```python
from build123d import *

# Parameters (mm, degrees)
SZKIC1_R                    = 2
DODANIE_WYCI_GNI_CIE1_DEPTH = 5
ZAOKR_GLENIE1_R             = 2
ZAOKR_GLENIE2_R             = 8


with BuildPart() as part:
    # Szkic1 → Dodanie-wyciągnięcie1 (new body)
    with BuildSketch(Plane.XY):
        with BuildLine():
            ThreePointArc((12, 0), (15, 3), (18, 0))
            Line((18, 0), (18, -15))
            Line((18, -15), (25, -15))
            Line((25, -15), (25, 15))
            Line((25, 15), (2, 15))
            Line((2, 15), (-2, 15))
            Line((-2, 15), (-25, 15))
            Line((-25, 15), (-25, -15))
            Line((-25, -15), (-18, -15))
            Line((-18, -15), (-18, 0))
            ThreePointArc((-18, 0), (-15, 3), (-12, 0))
            Line((-12, 0), (-12, -15))
            Line((-12, -15), (12, -15))
            Line((12, -15), (12, 0))
        make_face()
        with BuildLine():
            Line((-2, 15), (2, 15))
            Line((2, 15), (2, 20))
            ThreePointArc((2, 20), (0, 18), (-2, 20))
            Line((-2, 20), (-2, 15))
        make_face()
        with Locations((0, 20)):
            Circle(SZKIC1_R)
    extrude(amount=DODANIE_WYCI_GNI_CIE1_DEPTH)

    # Zaokrąglenie1
    zaokr_glenie1_edges = [part.edges().sort_by_distance(p)[0] for p in [
        (12, -15, 2.5),
        (-12, -15, 2.5),
        (-18, -15, 2.5),
        (-25, -15, 2.5),
        (-2, 15, 2.5),
        (2, 15, 2.5),
        (25, -15, 2.5),
        (18, -15, 2.5),
    ]]
    fillet(zaokr_glenie1_edges, radius=ZAOKR_GLENIE1_R)

    # Zaokrąglenie2
    zaokr_glenie2_edges = [part.edges().sort_by_distance(p)[0] for p in [
        (-25, 15, 2.5),
        (25, 15, 2.5),
    ]]
    fillet(zaokr_glenie2_edges, radius=ZAOKR_GLENIE2_R)


solid = part.part
```
Here's how the part is built. I have some questions about the finished solid (model axes, mm). A direction names the side the tool comes from. Give positions to 0.01 mm unless a question says otherwise; leave off trailing zeros. Order: outer loops, then holes, each group sorted by start corner. A loop starts at its lowest first (then second) coordinate and runs counter-clockwise, first axis right, second up. Notation, with made-up numbers: (-19.5, 12) - (-15.5, 12) arc R16 cw to (-15.5, 37) - close; hole circle Ø6 at (44, 61). An arc over 180 degrees is marked (long way). Answer as a JSON object with one key per item and string values. Group by question number.
Item 1: For P1, Ø2.5, axis at y = 18.5, z = 3, coming from the +X side; P2, Ø1.5, axis at x = -4.5, z = 1, coming from the +Y side; P3, Ø2, axis at x = -12.5, z = 2.5, coming from the -Y side, each with a flat end and sliding along its axis, tell me the tip position at first contact or that it passes through.
Item 2: If we section it at B-B on z = 2.1: Please give me the cut outline in (x, y), and give its area (3 significant figures).
Item 3: If we section it at D-D on x = -15: Please give me the cut outline in (y, z).
Item 4: If we section it at C-C on x = 6: Please give me the cut outline in (y, z), and give its area (3 significant figures).
Item 5: Please list where these lines run through material, in increasing order: probe 1 along X at (y, z) = (-10, 0.95); probe 2 along X at (y, z) = (2, 4.45); probe 3 along Y at (x, z) = (4.5, 2.85).
Item 6: Which directions (+Z, -Z, +X, -X, +Y, -Y) give clear straight access to the entire face, cutting with the end or side of a thin tool? Please do faces 1 (the flat face through (-12, -6, 2)), 2 (the flat face through (0, -15, 2)), 3 (the flat face through (-2, 19, 2)), 4 (the flat face through (2, 18, 2)).
Item 7: If we section it at A-A on y = -2.5: Please give me the cut outline in (x, z).
Result set:
{
 "1": {"P1": "x = 2", "P2": "y = 15.02", "P3": "y = -14.32"},
 "2": {"outline": "(-25, -13) arc R2 ccw to (-23, -15) - (-20, -15) arc R2 ccw to (-18, -13) - (-18, 0) arc R3 cw to (-12, 0) - (-12, -13) arc R2 ccw to (-10, -15) - (10, -15) arc R2 ccw to (12, -13) - (12, 0) arc R3 cw to (18, 0) - (18, -13) arc R2 ccw to (20, -15) - (23, -15) arc R2 ccw to (25, -13) - (25, 7) arc R8 ccw to (17, 15) - (4, 15) arc R2 cw to (2, 17) - (2, 20) arc R2 ccw to (-2, 20) - (-2, 17) arc R2 cw to (-4, 15) - (-17, 15) arc R8 ccw to (-25, 7) - close", "area": "1,290 mm²"},
 "3": {"outline": "(3, 0) - (15, 0) - (15, 5) - (3, 5) - close"},
 "4": {"outline": "(-15, 0) - (15, 0) - (15, 5) - (-15, 5) - close", "area": "150 mm²"},
 "5": {"probe 1": "-25 to -18, -12 to 12, 18 to 25", "probe 2": "-25 to -17.24, -12.76 to 12.76, 17.24 to 25", "probe 3": "-15 to 15"},
 "6": {"face 1": "+Z, -Z, -Y", "face 2": "+Z, -Z, +X, -X, -Y", "face 3": "+Z, -Z, -X, +Y", "face 4": "+Z, -Z, +X, +Y"},
 "7": {"outline": "(-25, 0) - (-18, 0) - (-18, 5) - (-25, 5) - close; (-12, 0) - (12, 0) - (12, 5) - (-12, 5) - close; (18, 0) - (25, 0) - (25, 5) - (18, 5) - close"}
}
